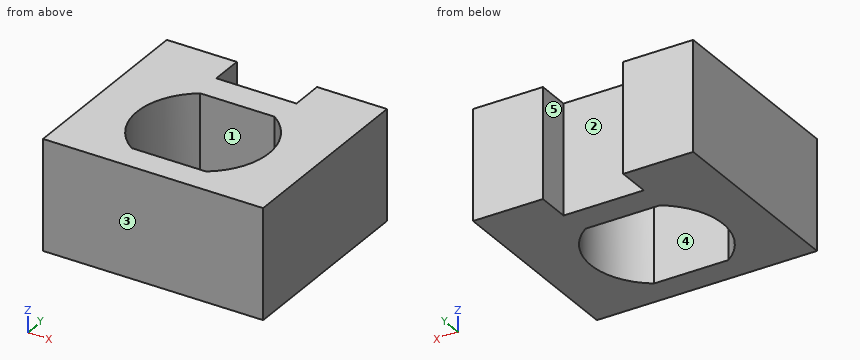
```python
from build123d import *

# Parameters (mm, degrees)
BOSS_EXTRUDE1_DEPTH = 10


with BuildPart() as part:
    # Sketch1 → Boss-Extrude1 (new body)
    with BuildSketch(Plane.XY):
        Polygon((0, 15.0114), (0, 0), (20.066, 0), (20.066, 15.0114), (20.066, 18.0086), (13.6884, 18.0086), (13.6884, 15.0114), (6.3776, 15.0114), (6.3776, 17.998004192), (0, 17.998004192), align=None)
        with BuildLine():
            Line((6.5532, 12.3952), (9.9441, 12.3952))
            Line((9.9441, 12.3952), (13.335, 12.3952))
            ThreePointArc((13.335, 12.3952), (15.967609722, 7.4168), (13.335, 2.4384))
            Line((13.335, 2.4384), (9.9441, 2.4384))
            Line((9.9441, 2.4384), (6.5532, 2.4384))
            ThreePointArc((6.5532, 2.4384), (3.920590278, 7.4168), (6.5532, 12.3952))
        make_face(mode=Mode.SUBTRACT)
    extrude(amount=BOSS_EXTRUDE1_DEPTH)


solid = part.part
```
Input: part model. Units: mm. Frame: model coordinates. Face numbers are marked on the shaded views. A direction names the side the tool comes from. Give positions to 0.01 mm unless a question says otherwise; leave off trailing zeros. Loops run counter-clockwise (first coordinate to the right, second up) from the corner with the lowest first, then second, coordinate; pieces in that order, holes last. Notation, with made-up numbers: (20.5, -10.5) -> (70.5, -10.5) arc R26 ccw to (70.5, 18.5) -> close; hole circle Ø1 at (32, 23). An arc over 180 degrees is marked (long way). Use a Markdown table: item, result.
Q1. Pull-direction query (Y, two-part tool) for the marked faces 1, 2 and 3; classes: pulls with the +Y half, pulls with the -Y half, needs draft (parallel to the pull), parting line crosses it, or undercut.
Entries:
| item | result |
|---|---|
| face 1 | undercut |
| face 2 | pulls with the +Y half |
| face 3 | pulls with the -Y half |
Q2. Section query A-A, the plane x = 10.25. Return the cut outline in (y, z).
Entries:
| item | result |
|---|---|
| outline | (0, 0) -> (2.44, 0) -> (2.44, 10) -> (0, 10) -> close; (12.4, 0) -> (15.01, 0) -> (15.01, 10) -> (12.4, 10) -> close |
Q3. First-contact query: P1, Ø6, axis at x = 2, z = 2.5, coming from the +Y side; P2, Ø6, axis at x = 10.5, z = 5.5, coming from the +Y side. Flat tips, straight axial feed; report the tip coordinate or a pass-through.
Entries:
| item | result |
|---|---|
| P1 | stops at y = 18 |
| P2 | stops at y = 15.01 |
Q4. Ray query, probe 1 along X at (y, z) = (15.5, 3.25); probe 2 along Y at (x, z) = (8.25, 6); probe 3 along Y at (x, z) = (2.25, 3.75). Return the intervals inside material, ascending. Write a range as from..to.
Entries:
| item | result |
|---|---|
| probe 1 | x = 0..6.38, 13.69..20.07 |
| probe 2 | y = 0..2.44, 12.4..15.01 |
| probe 3 | y = 0..18 |
Q5. Section query C-C, the plane z = 6.5. Return the cut outline in (x, y) (1 decimal), plus the area to 3 significant figures.
Entries:
| item | result |
|---|---|
| outline | (0, 0) -> (20.1, 0) -> (20.1, 18) -> (13.7, 18) -> (13.7, 15) -> (6.4, 15) -> (6.4, 18) -> (0, 18) -> close; hole (6.6, 2.4) -> (13.3, 2.4) arc R6 ccw to (13.3, 12.4) -> (6.6, 12.4) arc R6 ccw to start |
| area | 235 mm² |
Q6. Section query B-B, the plane y = 16.5. Return the cut outline in (x, z).
Entries:
| item | result |
|---|---|
| outline | (0, 0) -> (6.38, 0) -> (6.38, 10) -> (0, 10) -> close; (13.69, 0) -> (20.07, 0) -> (20.07, 10) -> (13.69, 10) -> close |
Q7. Access query for the marked faces 4 and 5. Directions: +Z, -Z, +X, -X, +Y, -Y. A direction counts if a zero-diameter tool reaches every point of the face in a straight line with its end or side. Return the directions, or none.
Entries:
| item | result |
|---|---|
| face 4 | +Z, -Z |
| face 5 | +Z, -Z, +Y |
